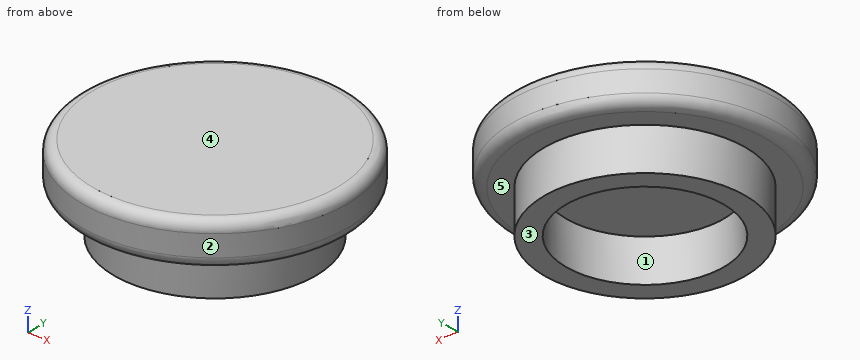
```python
from build123d import *

# Parameters (mm, degrees)
F0_R     = 15.875
F0_R_2   = 12.065
F0_R_3   = 9.45129
F1_DEPTH = 5.08
F2_DEPTH = 5.08
F3_R     = 1.27


with BuildPart() as f1:
    # F0 (on Top) → F1 (new body)
    with BuildSketch(Plane.XY):
        Circle(F0_R)
        Circle(F0_R_2, mode=Mode.SUBTRACT)
        Circle(F0_R_2)
        Circle(F0_R_3, mode=Mode.SUBTRACT)
        Circle(F0_R_3)
    extrude(amount=F1_DEPTH)

    # F0 (on Top) → F2 (join)
    with BuildSketch(Plane.XY):
        Circle(F0_R_2)
        Circle(F0_R_3, mode=Mode.SUBTRACT)
    extrude(amount=-F2_DEPTH)

    # F3
    f3_edges = [f1.edges().sort_by_distance(p)[0] for p in [
        (-15.875, 0, 5.08),
        (-15.875, 0, 0),
    ]]
    fillet(f3_edges, radius=F3_R)


solid = f1.part
```
Check sheet for the modelled part. Datum: model origin and axes. Units: mm. Face numbers are marked on the shaded views. A direction names the side the tool comes from. Give positions to 0.01 mm unless a question says otherwise; leave off trailing zeros. Write each loop counter-clockwise with the first axis right and the second up, starting at its lowest first coordinate (ties: lowest second). Pieces come first, ordered by that corner, then holes. Notation, with made-up numbers: (36, 88.5) -> (42, 88.5) arc R8 ccw to (42, 103.5) -> close; hole circle Ø10 at (67.5, 51.25). An arc over 180 degrees is marked (long way). Use CSV: the item, a comma, the result in double quotes. Start each with the question number.
Q1. Cross-section at C-C on z = 2.5. Enter the section's corners in (x, y) (3 decimals).
Q2. Release check for a two-part mould opening along X. For the marked faces 1, 2 and 3 record: +X half, -X half, draft (parallel to the pull), parting line (faces both ways), or undercut.
Q3. Depth check by flat-ended pin: P1, Ø9.5, axis at x = -2.5, y = -1, coming from the -Z side; P2, Ø5, axis at x = 12.5, z = 2.5, coming from the -Y side; P3, Ø1, axis at y = 8.5, z = 0, coming from the -X side. Enter the tip coordinate at first touch or a pass-through.
Q4. Tool access check on the marked faces 4 and 5. Record the directions out of +Z, -Z, +X, -X, +Y, -Y that give a thin tool (end or side, any length) a straight path to the whole face; none if there is none.
Q5. Scan lines: line 1 along Y through (x, z) = (0, -3.5) (3 decimals); line 2 along Z through (x, y) = (5.5, -6.5); line 3 along X through (y, z) = (8, -0.5). Record each from-to range of solid material in increasing order.
Q6. Cross-section at A-A on y = 0. Enter the section's corners in (x, z) (3 decimals).
Working result:
1,outline,"circle Ø31.75 at (0, 0)"
2,face 1,"undercut"
2,face 2,"parting line"
2,face 3,"draft"
3,P1,"stops at z = 0"
3,P2,"stops at y = -12.33"
3,P3,"stops at x = -13.19"
4,face 4,"+Z, +X, -X, +Y, -Y"
4,face 5,"-Z"
5,line 1,"y = -12.065 to -9.451, 9.451 to 12.065"
5,line 2,"z = 0 to 5.08"
5,line 3,"x = -9.03 to -5.03, 5.03 to 9.03"
6,outline,"(-15.875, 1.27) arc R1.27 ccw to (-14.605, 0) -> (-12.065, 0) -> (-12.065, -5.08) -> (-9.451, -5.08) -> (-9.451, 0) -> (9.451, 0) -> (9.451, -5.08) -> (12.065, -5.08) -> (12.065, 0) -> (14.605, 0) arc R1.27 ccw to (15.875, 1.27) -> (15.875, 3.81) arc R1.27 ccw to (14.605, 5.08) -> (-14.605, 5.08) arc R1.27 ccw to (-15.875, 3.81) -> close"
